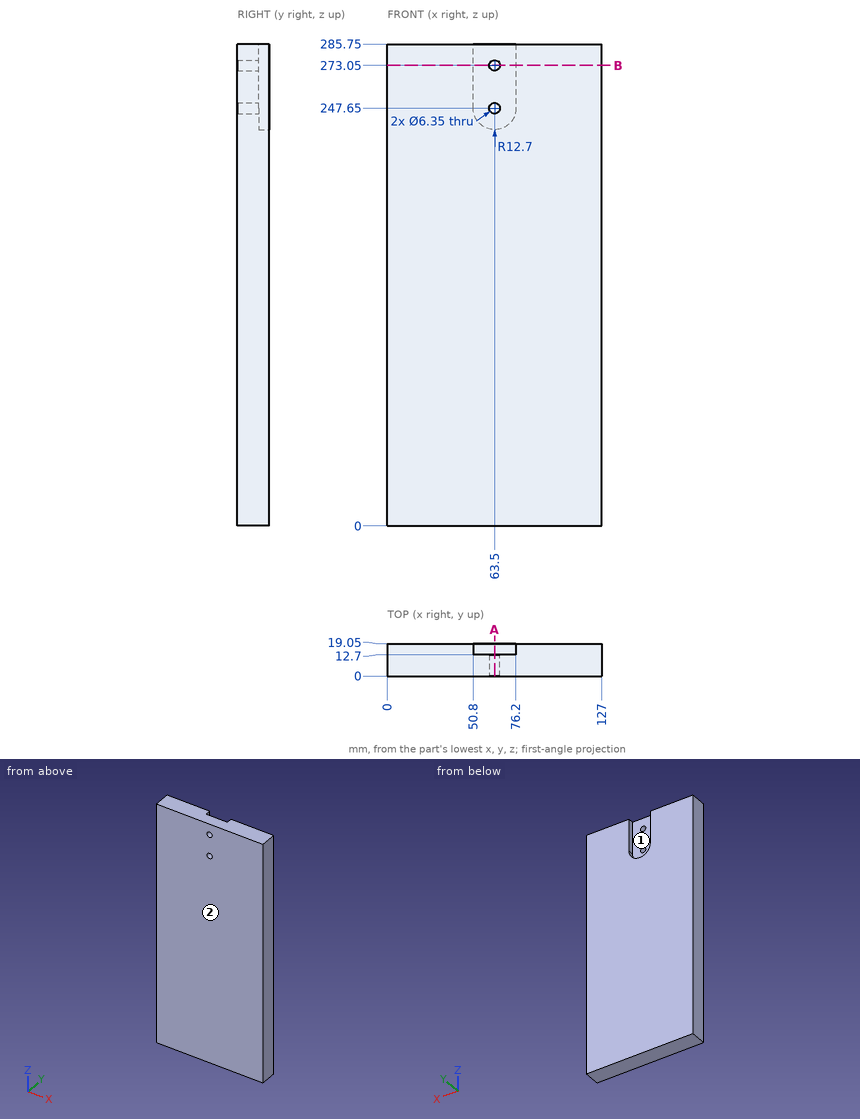
The drawing under review shows one solid part. Ordinate dimensions are in mm from its lowest x, y, z. A direction names the side the tool comes from. Give positions to 0.01 mm unless a question says otherwise; leave off trailing zeros. Loops run counter-clockwise (first coordinate to the right, second up) from the corner with the lowest first, then second, coordinate; pieces in that order, holes last. Notation, with made-up numbers: M 56.5,9 L 83.5,9 A15 cw 83.5,37 Z; hole C 40.25,-33.5 d1. An arc over 180 degrees is marked long. One line per question, with ' | ' between items. Start each with the question number.
1. Add section B-B (z = 273.05). Write out the cut boundary in (x, y) (3 decimals).
2. For the marked faces 1 and 2, list the 3-axis set-ups (+Z, -Z, +X, -X, +Y, -Y) from which the entire face can be reached by the end or side of a thin tool; tool diameter is ignored.
3. Add section A-A (x = 63.5). Write out the cut boundary in (y, z) (3 decimals).
4. To check wall thickness, follow L1, parallel to Z at x = 63.5, y = 4.5 (3 decimals); L2, parallel to X at y = 6.75, z = 273.05 (3 decimals). State the ranges of each line that lie inside material, in increasing order.
Worked out:
1) outline: M 0,0 L 60.325,0 L 60.325,12.7 L 50.8,12.7 L 50.8,19.05 L 0,19.05 Z; M 66.675,0 L 127,0 L 127,19.05 L 76.2,19.05 L 76.2,12.7 L 66.675,12.7 Z
2) face 1: +Z, +Y | face 2: +Z, -Z, +X, -X, -Y
3) outline: M 0,0 L 19.05,0 L 19.05,234.95 L 12.7,234.95 L 12.7,244.475 L 0,244.475 Z; M 0,250.825 L 12.7,250.825 L 12.7,269.875 L 0,269.875 Z; M 0,276.225 L 12.7,276.225 L 12.7,285.75 L 0,285.75 Z
4) L1: z = 0 to 244.475, 250.825 to 269.875, 276.225 to 285.75 | L2: x = 0 to 60.325, 66.675 to 127
